```python
from build123d import *

# Parameters (mm, degrees)
F2_R     = 0.3
F3_SIZE2 = 0.5
F3_SIZE  = 0.5
F4_W     = 4
F4_H     = 6
F5_DEPTH = 3.5
F6_SIZE2 = 0.2
F6_SIZE  = 0.2


with BuildPart() as f1:
    # F0 (on Front) → F1 (revolve)
    with BuildSketch(Plane.XZ):
        Polygon((0, 62.1), (0, 0), (3.875, 0), (3.875, 5), (4, 5), (4, 42.7), (3.025, 42.7), (3.025, 62.1), align=None)
    revolve(axis=Axis((0, 0, 31.05), (0, 0, 1)))

    # F2
    f2_edges = [f1.edges().sort_by_distance(p)[0] for p in [
        (-3.025, 0, 42.7),
    ]]
    fillet(f2_edges, radius=F2_R)

    # F3
    f3_edges = [f1.edges().sort_by_distance(p)[0] for p in [
        (-3.875, 0, 0),
    ]]
    chamfer(f3_edges, length=F3_SIZE, length2=F3_SIZE2)

    # F4 (on face) → F5 (cut)
    with BuildSketch(Plane.XY.offset(62.1)):
        with Locations((-4, 0)):
            Rectangle(F4_W, F4_H)
        with Locations((4, 0)):
            Rectangle(F4_W, F4_H)
    extrude(amount=-F5_DEPTH, mode=Mode.SUBTRACT)

    # F6
    f6_edges = [f1.edges().sort_by_distance(p)[0] for p in [
        (2, 0, 62.1),
        (0, 3.025, 62.1),
        (0, -3.025, 62.1),
        (-2, 0, 62.1),
    ]]
    chamfer(f6_edges, length=F6_SIZE, length2=F6_SIZE2)


solid = f1.part
```
Can you work these out from the model? Positions are in its coordinate system, mm. A direction names the side the tool comes from. Coordinates: 2 decimals unless noted, no trailing zeros. Loops run counter-clockwise (first coordinate to the right, second up) from the corner with the lowest first, then second, coordinate; pieces in that order, holes last. Notation, with made-up numbers: (14.5, 21.25) -> (47.5, 21.25) arc R18 cw to (47.5, 26.25) -> close; hole circle Ø8 at (46.25, 58.5). An arc over 180 degrees is marked (long way). Answer as a JSON object with one key per item and string values.
1) Imagine slicing it at A-A (y = 0). Please give me the cut outline in (x, z) (3 decimals), then the cut area to 3 significant figures.
Results:
{"outline": "(-4, 5) -> (-3.875, 5) -> (-3.875, 0.5) -> (-3.375, 0) -> (3.375, 0) -> (3.875, 0.5) -> (3.875, 5) -> (4, 5) -> (4, 42.7) -> (3.325, 42.7) arc R0.3 cw to (3.025, 43) -> (3.025, 58.6) -> (2, 58.6) -> (2, 61.9) -> (1.8, 62.1) -> (-1.8, 62.1) -> (-2, 61.9) -> (-2, 58.6) -> (-3.025, 58.6) -> (-3.025, 43) arc R0.3 cw to (-3.325, 42.7) -> (-4, 42.7) -> close", "area": "450 mm^2"}
2) For P1, Ø4, axis at y = 1, z = 49, coming from the +X side (3 decimals); P2, Ø4, axis at x = -3, z = 14.5, coming from the +Y side; P3, Ø1, axis at y = -3, z = 55, coming from the +X side, each with a flat end and sliding along its axis, tell me the tip position at first contact or that it passes through.
Results:
{"P1": "stops at x = 3.025", "P2": "stops at y = 3.87", "P3": "stops at x = 1.7"}
3) If I drill on line 1 (X direction, y = 1, z = 8); line 2 (X direction, y = -0.25, z = 8); line 3 (Y direction, x = -2.25, z = 57), over which ranges is the centre line in solid material (lowest first)?
Results:
{"line 1": "x = -3.87 to 3.87", "line 2": "x = -3.99 to 3.99", "line 3": "y = -2.02 to 2.02"}
4) Imagine slicing it at C-C (z = 30). Please give me the cut outline in (x, y).
Results:
{"outline": "circle Ø8 at (0, 0)"}
5) Imagine slicing it at B-B (x = 0). Please give me the cut outline in (y, z) (3 decimals).
Results:
{"outline": "(-4, 5) -> (-3.875, 5) -> (-3.875, 0.5) -> (-3.375, 0) -> (3.375, 0) -> (3.875, 0.5) -> (3.875, 5) -> (4, 5) -> (4, 42.7) -> (3.325, 42.7) arc R0.3 cw to (3.025, 43) -> (3.025, 61.9) -> (2.825, 62.1) -> (-2.825, 62.1) -> (-3.025, 61.9) -> (-3.025, 43) arc R0.3 cw to (-3.325, 42.7) -> (-4, 42.7) -> close"}
6) For faces 1 (the face through (-2, 0, 60)), 2 (the face through (-2, 3, 42.7)), 3 (the face through (-0.504, 3.842, 2.782)), 4 (the face through (2, 0, 60)), which set-ups out of +Z, -Z, +X, -X, +Y, -Y let a thin tool reach every point of the face, with its end or its side?
Results:
{"face 1": "+Z, -X, +Y, -Y", "face 2": "+Z", "face 3": "-Z", "face 4": "+Z, +X, +Y, -Y"}
